For this review, take the finished solid that the model builds, in its own axes (mm). Round coordinates to 2 decimals unless told otherwise and drop trailing zeros.
1. To check wall thickness, follow line 1 along X through (y, z) = (-7.25, 244); line 2 along Y through (x, z) = (-7.5, 341); line 3 along Y through (x, z) = (0, 227.5). State the ranges of each line that lie inside material, in increasing order.
2. Consider section A-A on z = 445. State how many separate pieces and enclosed holes the cut face has, then the cut area to 3 significant figures.
3. Clearance check with flat-ended pins moving along their axes: pin 1 Ø1.8 at (y, z) = (0, 256) entering from -X; pin 2 Ø3 at (y, z) = (-1, 288) entering from +X; pin 3 Ø1.5 at (x, z) = (18, 162.5) entering from +Y; pin 4 Ø2 at (x, y) = (-11.5, 3.5) entering from -Z. State where each tip first meets the part, or that it passes through.
from build123d import *

# Parameters (mm, degrees)
SKETCH_1_R      = 2.5
EXTRUDE_2_DEPTH = 600


with BuildPart() as part:
    # 草图1 → 凸台-拉伸2 (new body)
    with BuildSketch(Plane.XY):
        with BuildLine():
            Line((-23.2, 10), (-28, 10))
            ThreePointArc((-28, 10), (-29.414213562, 9.414213562), (-30, 8))
            Line((-30, 8), (-30, 3.2))
            Line((-30, 3.2), (-28, 3.2))
            Line((-28, 3.2), (-28, 5.5))
            Line((-28, 5.5), (-26.5, 5.5))
            Line((-26.5, 5.5), (-23.9, 3))
            Line((-23.9, 3), (-23.9, -3))
            Line((-23.9, -3), (-26.5, -5.5))
            Line((-26.5, -5.5), (-28, -5.5))
            Line((-28, -5.5), (-28, -3.2))
            Line((-28, -3.2), (-30, -3.2))
            Line((-30, -3.2), (-30, -8.5))
            ThreePointArc((-30, -8.5), (-29.560660172, -9.560660172), (-28.5, -10))
            Line((-28.5, -10), (-23.2, -10))
            Line((-23.2, -10), (-23.2, -8))
            Line((-23.2, -8), (-25.5, -8))
            Line((-25.5, -8), (-25.5, -6.5))
            Line((-25.5, -6.5), (-23, -3.9))
            Line((-23, -3.9), (-17, -3.9))
            Line((-17, -3.9), (-14.5, -6.5))
            Line((-14.5, -6.5), (-14.5, -8))
            Line((-14.5, -8), (-16.8, -8))
            Line((-16.8, -8), (-16.8, -10))
            Line((-16.8, -10), (-3.2, -10))
            Line((-3.2, -10), (-3.2, -8))
            Line((-3.2, -8), (-5.5, -8))
            Line((-5.5, -8), (-5.5, -6.5))
            Line((-5.5, -6.5), (-3, -3.9))
            Line((-3, -3.9), (3, -3.9))
            Line((3, -3.9), (5.5, -6.5))
            Line((5.5, -6.5), (5.5, -8))
            Line((5.5, -8), (3.2, -8))
            Line((3.2, -8), (3.2, -10))
            Line((3.2, -10), (16.8, -10))
            Line((16.8, -10), (16.8, -8))
            Line((16.8, -8), (14.5, -8))
            Line((14.5, -8), (14.5, -6.5))
            Line((14.5, -6.5), (17, -3.9))
            Line((17, -3.9), (23, -3.9))
            Line((23, -3.9), (25.5, -6.5))
            Line((25.5, -6.5), (25.5, -8))
            Line((25.5, -8), (23.2, -8))
            Line((23.2, -8), (23.2, -10))
            Line((23.2, -10), (28.5, -10))
            ThreePointArc((28.5, -10), (29.560660172, -9.560660172), (30, -8.5))
            Line((30, -8.5), (30, -3.2))
            Line((30, -3.2), (28, -3.2))
            Line((28, -3.2), (28, -5.5))
            Line((28, -5.5), (26.5, -5.5))
            Line((26.5, -5.5), (23.9, -3))
            Line((23.9, -3), (23.9, 3))
            Line((23.9, 3), (26.5, 5.5))
            Line((26.5, 5.5), (28, 5.5))
            Line((28, 5.5), (28, 3.2))
            Line((28, 3.2), (30, 3.2))
            Line((30, 3.2), (30, 8.5))
            ThreePointArc((30, 8.5), (29.560660172, 9.560660172), (28.5, 10))
            Line((28.5, 10), (23.2, 10))
            Line((23.2, 10), (23.2, 8))
            Line((23.2, 8), (25.5, 8))
            Line((25.5, 8), (25.5, 6.5))
            Line((25.5, 6.5), (23, 3.9))
            Line((23, 3.9), (17, 3.9))
            Line((17, 3.9), (14.5, 6.5))
            Line((14.5, 6.5), (14.5, 8))
            Line((14.5, 8), (16.8, 8))
            Line((16.8, 8), (16.8, 10))
            Line((16.8, 10), (3.2, 10))
            Line((3.2, 10), (3.2, 8))
            Line((3.2, 8), (5.5, 8))
            Line((5.5, 8), (5.5, 6.5))
            Line((5.5, 6.5), (3, 3.9))
            Line((3, 3.9), (-3, 3.9))
            Line((-3, 3.9), (-5.5, 6.5))
            Line((-5.5, 6.5), (-5.5, 8))
            Line((-5.5, 8), (-3.2, 8))
            Line((-3.2, 8), (-3.2, 10))
            Line((-3.2, 10), (-16.8, 10))
            Line((-16.8, 10), (-16.8, 8))
            Line((-16.8, 8), (-14.5, 8))
            Line((-14.5, 8), (-14.5, 6.5))
            Line((-14.5, 6.5), (-17, 3.9))
            Line((-17, 3.9), (-23, 3.9))
            Line((-23, 3.9), (-25.5, 6.5))
            Line((-25.5, 6.5), (-25.5, 8))
            Line((-25.5, 8), (-23.2, 8))
            Line((-23.2, 8), (-23.2, 10))
        make_face()
        Polygon((-12.75, -8), (-12.75, -5.5), (-13.5, -5.5), (-16.1, -3), (-16.1, 3), (-13.5, 5.5), (-12.75, 5.5), (-12.75, 8), (-7.25, 8), (-7.25, 5.5), (-6.5, 5.5), (-3.9, 3), (-3.9, -3), (-6.5, -5.5), (-7.25, -5.5), (-7.25, -8), align=None, mode=Mode.SUBTRACT)
        Polygon((6.5, -5.5), (3.9, -3), (3.9, 3), (6.5, 5.5), (7.25, 5.5), (7.25, 8), (12.75, 8), (12.75, 5.5), (13.5, 5.5), (16.1, 3), (16.1, -3), (13.5, -5.5), (12.75, -5.5), (12.75, -8), (7.25, -8), (7.25, -5.5), align=None, mode=Mode.SUBTRACT)
        with Locations((20, 0)):
            Circle(SKETCH_1_R, mode=Mode.SUBTRACT)
        with Locations((-20, 0)):
            Circle(SKETCH_1_R, mode=Mode.SUBTRACT)
        Circle(SKETCH_1_R, mode=Mode.SUBTRACT)
    extrude(amount=EXTRUDE_2_DEPTH)


solid = part.part
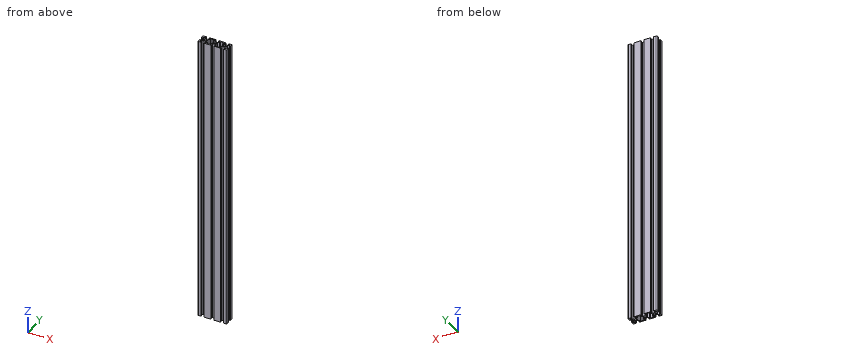
Resolved:
1. line 1: x = -30 to -25.5, -14.5 to -12.75, -7.25 to -5.5, 5.5 to 7.25, 12.75 to 14.5, 25.5 to 30
1. line 2: y = -10 to -8, 8 to 10
1. line 3: y = -3.9 to -2.5, 2.5 to 3.9
2. separate pieces: 1
2. enclosed holes: 5
2. area: 430 mm2
3. pin 1: stops at x = -23.9
3. pin 2: stops at x = 23.9
3. pin 3: stops at y = 3.9
3. pin 4: passes through
